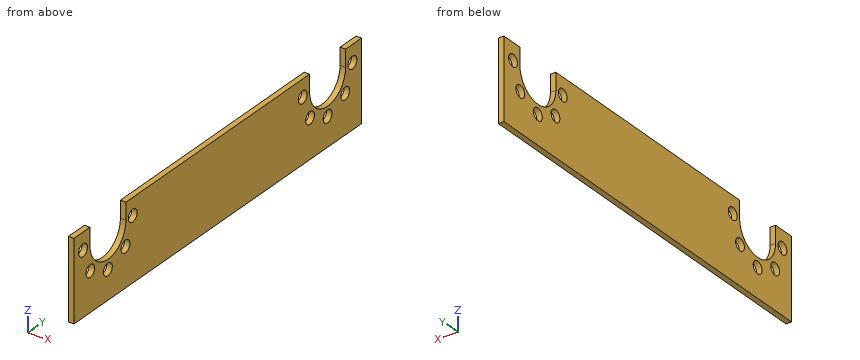
from build123d import *

# Parameters (mm, degrees)
F0_W     = 1
F0_H     = 20
F1_DEPTH = 72
F2_R     = 1.1
F3_DEPTH = 1.001
F4_W     = 72
F4_H     = 5.4
F5_DEPTH = 1.001


with BuildPart() as f1:
    # F0 (on Front) → F1 (new body)
    with BuildSketch(Plane.XZ):
        with Locations((-0.5, 10)):
            Rectangle(F0_W, F0_H)
    extrude(amount=F1_DEPTH)

    # F2 (on face) → F3 (cut, through all)
    with BuildSketch(Plane(origin=(-1, 0, 0), x_dir=(0, -1, 0), z_dir=(-1, 0, 0))):
        with BuildLine():
            Line((4, 20), (4, 11.5))
            ThreePointArc((4, 11.5), (8.5, 7), (13, 11.5))
            Line((13, 11.5), (13, 20))
            Line((13, 20), (4, 20))
        make_face()
        with Locations((2.27746, 11.5)):
            Circle(F2_R)
        with Locations((4.1, 7.1)):
            Circle(F2_R)
        with Locations((8.5, 5.27746)):
            Circle(F2_R)
        with Locations((12.9, 7.1)):
            Circle(F2_R)
        with Locations((14.72254, 11.5)):
            Circle(F2_R)
        with BuildLine():
            ThreePointArc((59, 11.5), (63.5, 7), (68, 11.5))
            Line((68, 11.5), (68, 20))
            Line((68, 20), (59, 20))
            Line((59, 20), (59, 11.5))
        make_face()
        with Locations((69.72254, 11.5)):
            Circle(F2_R)
        with Locations((67.9, 7.1)):
            Circle(F2_R)
        with Locations((63.5, 5.27746)):
            Circle(F2_R)
        with Locations((59.1, 7.1)):
            Circle(F2_R)
        with Locations((57.27746, 11.5)):
            Circle(F2_R)
    extrude(amount=-F3_DEPTH, mode=Mode.SUBTRACT)

    # F4 (on face) → F5 (cut, through all)
    with BuildSketch(Plane(origin=(-1, 0, 0), x_dir=(0, -1, 0), z_dir=(-1, 0, 0))):
        with Locations((36, 17.3)):
            Rectangle(F4_W, F4_H)
    extrude(amount=-F5_DEPTH, mode=Mode.SUBTRACT)


solid = f1.part
Part model, mm, in its own coordinate system. Coordinates: 2 decimals unless noted, no trailing zeros. Order: outer loops, then holes, each group sorted by start corner. A loop starts at its lowest first (then second) coordinate and runs counter-clockwise, first axis right, second up.
(1) Slice it at B-B, the plane x = -0.8. State how many separate pieces and enclosed holes the cut face has, and give its area (3 significant figures).
Check sheet entries:
separate pieces: 1
enclosed holes: 10
area: 894 mm2
(2) Slice it at A-A, the plane y = -8.5. Write the cut outline in (x, z).
Check sheet entries:
outline: (-1, 0) - (0, 0) - (0, 4.18) - (-1, 4.18) - close; (-1, 6.38) - (0, 6.38) - (0, 7) - (-1, 7) - close
(3) Pin check, flat tip, straight feed: pin 1 Ø2 at (y, z) = (-57.28, 11.5) entering from -X. Stop position of the tip, or through.
Check sheet entries:
pin 1: passes through
(4) Probe L1, parallel to Y at x = -0.15, z = 13; L2, parallel to Y at x = -0.8, z = 4.5; L3, parallel to Z at x = -0.4, y = -9. List the from-to ranges inside material, lowest first.
Check sheet entries:
L1: y = -72 to -68, -59 to -13, -4 to 0
L2: y = -72 to -64.28, -62.72 to -9.28, -7.72 to 0
L3: z = 0 to 4.3, 6.26 to 7.03
